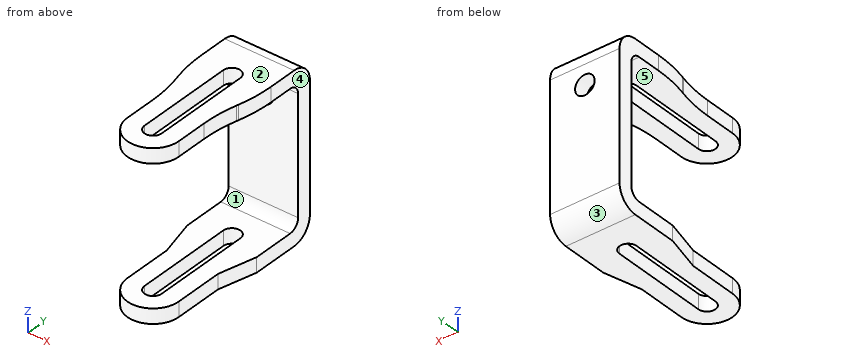
Autodesk Inventor part; units mm, degrees
ref_plane "YZ Plane" through (0, 0, 0) normal (1, 0, 0) x (0, 1, 0)
ref_plane "XZ Plane" through (0, 0, 0) normal (0, 1, 0) x (-1, 0, 0)
ref_plane "XY Plane" through (0, 0, 0) normal (0, 0, 1) x (1, 0, 0)
sketch "Sketch1" plane through (0, 0, 0) normal (0, 1, 0) x (-1, 0, 0)
  line L0 (7.1, -17) -> (-7.1, -17)
  line L1 (-7.1, -17) -> (-7.1, 17)
  line L2 (-7.1, 17) -> (7.1, 17)
  line L3 (7.1, 17) -> (7.1, -17)
  line L4 (7.1, -17) -> (-7.1, 17) construction
  line L5 (-7.1, -17) -> (7.1, 17) construction
  circle A0 centre (0, 9) radius 2
  point P0 (0, 0)
  dimension "d0" = 14.2
  dimension "d1" = 34
  dimension "d4" = 4
  dimension "d5" = 8
  dimension "d6" = 7.1
extrude "Extrusion1" add sketch "Sketch1" along normal blind 3
sketch "Sketch2" plane through (-7.1, 0, 17) normal (0, 0, 1) x (1, 0, 0)
  line L0 (7.1, -28) -> (7.1, -8) construction
  line L1 (8.85, -28) -> (8.85, -8)
  line L2 (5.35, -8) -> (5.35, -28)
  arc A0 (5.35, -28) -> (8.85, -28) centre (7.1, -28) ccw
  arc A1 (8.85, -8) -> (5.35, -8) centre (7.1, -8) ccw
  line L3 (0, 0) -> (0, 3)
  line L4 (0, 0) -> (14.2, 0)
  line L5 (1.85, -28) -> (1.85, -8)
  arc A2 (12.35, -8) -> (1.85, -8) centre (7.1, -8) ccw
  line L6 (12.35, -8) -> (12.35, -28)
  arc A3 (1.85, -28) -> (12.35, -28) centre (7.1, -28) ccw
  line L7 (0, 0) -> (0, -10.5)
  line L8 (0, -10.5) -> (1.85, -18)
  line L9 (14.2, 0) -> (14.2, -10.5)
  line L10 (14.2, -10.5) -> (12.35, -18)
  point P0 (7.1, 0)
  point P1 (7.1, -18)
  point P2 (8.85, -18)
  dimension "d7" = 7.1
  dimension "d8" = 3.5
  dimension "d9" = 20
  dimension "d10" = 18
  dimension "d11" = 3.5
extrude "Extrusion2" add sketch "Sketch2" against normal blind 3
fillet "Fillet1" radius 30 4 edges at (7.1, -10.5, 15.5) (5.25, -18, 15.5) (-7.1, -10.5, 15.5) (-5.25, -18, 15.5)
mirror "Mirror1" about plane through (0, 0, 0) normal (0, 0, 1) of "Extrusion2"
fillet "Fillet2" radius 4 2 edges at (0, 3, 17) (0, 3, -17)
fillet "Fillet3" radius 2 2 edges at (0, 0, 14) (0, 0, -14)
properties part number "SoporteSensorDeInterrupciones"
Can you work these out from the model? Positions are in its coordinate system, mm. Face numbers are marked on the shaded views. A direction names the side the tool comes from. Give positions to 0.01 mm unless a question says otherwise; leave off trailing zeros. Order: outer loops, then holes, each group sorted by start corner. A loop starts at its lowest first (then second) coordinate and runs counter-clockwise, first axis right, second up. Notation, with made-up numbers: M 41,71.5 L 77,71.5 A36 cw 77,108.5 Z; hole C 37,65 d1. An arc over 180 degrees is marked long. One line per item, written item: value.
1) I want a section at D-D, the plane x = 4.25. List the corners of the cut face in (y, z) for me.
Answer sheet:
outline: M -31.08,-17 L -1,-17 A4 ccw 3,-13 L 3,13 A4 ccw -1,17 L -31.08,17 L -31.08,14 L -2,14 A2 cw 0,12 L 0,-12 A2 cw -2,-14 L -31.08,-14 Z
2) We'd pull the mould along Z, two halves only. Please class the marked faces 3, 4 and 5: released by +Z, released by -Z, zero draft, split by the parting line, or undercut.
Answer sheet:
face 3: released by -Z
face 4: zero draft
face 5: undercut
3) I want a section at B-B, the plane x = 0. List the corners of the cut face in (y, z) for me, plus the area to 3 significant figures.
Answer sheet:
outline: M -33.25,-17 L -29.75,-17 L -29.75,-14 L -33.25,-14 Z; M -33.25,14 L -29.75,14 L -29.75,17 L -33.25,17 Z; M -6.25,-17 L -1,-17 A4 ccw 3,-13 L 3,7 L 0,7 L 0,-12 A2 cw -2,-14 L -6.25,-14 Z; M -6.25,14 L -2,14 A2 cw 0,12 L 0,11 L 3,11 L 3,13 A4 ccw -1,17 L -6.25,17 Z
area: 143 mm^2
4) Please list where these lines run through material, in increasing order: line 1 along Z through (x, y) = (6, -11.5); line 2 along Y through (x, z) = (-2.75, 4); line 3 along Z through (x, y) = (0, 1.8).
Answer sheet:
line 1: z = -17 to -14, 14 to 17
line 2: y = 0 to 3
line 3: z = -15.86 to 7, 11 to 15.86
5) For P1, Ø3.5, axis at y = -24, z = 16, coming from the +X side; P2, Ø1.5, axis at y = -21, z = -16, coming from the -X side; P3, Ø7, axis at x = -1.5, y = -17, coming from the -Z side; P4, Ø0.9, axis at y = -14, z = 16, coming from the +X side, each with a flat end and sliding along its axis, tell me the tip position at first contact or that it passes through.
Answer sheet:
P1: stops at x = 5.25
P2: stops at x = -5.25
P3: stops at z = -17
P4: stops at x = 6.34
6) On a 3-axis mill with a long thin cutter (end or side, diameter ignored), from which of +Z, -Z, +X, -X, +Y, -Y can I reach the whole of each face in a straight line? I mean the marked faces 1 and 2. Say none if no direction works.
Answer sheet:
face 1: +X, -X, -Y
face 2: +Z, +X, -X, +Y, -Y
7) I want a section at A-A, the plane y = -24. List the corners of the cut face in (x, z) for me, plus the area to 3 significant figures.
Answer sheet:
outline: M -5.25,-17 L -1.75,-17 L -1.75,-14 L -5.25,-14 Z; M -5.25,14 L -1.75,14 L -1.75,17 L -5.25,17 Z; M 1.75,-17 L 5.25,-17 L 5.25,-14 L 1.75,-14 Z; M 1.75,14 L 5.25,14 L 5.25,17 L 1.75,17 Z
area: 42.0 mm^2
8) I want a section at C-C, the plane z = 9. List the corners of the cut face in (x, y) for me.
Answer sheet:
outline: M -7.1,0 L -2,0 L -2,3 L -7.1,3 Z; M 2,0 L 7.1,0 L 7.1,3 L 2,3 Z
